Verification items for this drawing (mm, ordinates from the low corner). A direction names the side the tool comes from. Coordinates: 2 decimals unless noted, no trailing zeros. Order: outer loops, then holes, each group sorted by start corner. A loop starts at its lowest first (then second) coordinate and runs counter-clockwise, first axis right, second up. Notation, with made-up numbers: (-37.75, 13.5) -> (-13.75, 13.5) arc R19 ccw to (-13.75, 34.5) -> close; hole circle Ø9 at (-33, -40). An arc over 180 degrees is marked (long way). Write each question's results on one line, items separated by ' | '. Start each with the question number.
(1) Thickness scan on probe 1 along Y at (x, z) = (4.5, 7.7); probe 2 along X at (y, z) = (19, 7.7); probe 3 along Z at (x, y) = (2, 22.5). Record the ranges inside material, lowest first. Write a range as [from, to].
(2) Draft check along X on the marked faces 4, 5, 6 and 7. Enter one of: +X half, -X half, draft (parallel to the pull), parting line (faces both ways), or undercut.
(3) Cross-section at D-D on y = 19.75. Enter the section's corners in (x, z).
(4) Cross-section at C-C on z = 4.75. Enter the section's corners in (x, y), and give its area (3 significant figures).
(5) Cross-section at B-B on x = 30. Enter the section's corners in (y, z).
(6) Cross-section at A-A on z = 8. Enter the section's corners in (x, y), and give its area (3 significant figures).
(7) Go/stop test with flat-tipped pins: pin 1 (9 mm diameter, centred on x = 29.5, y = 18, fed in from -Z); pin 2 (10 mm diameter, centred on x = 11, y = 10.5, fed in from -Z); pin 3 (1.5 mm diameter, centred on y = 13.5, z = 5, fed in from +X). Record where each tip stops, or that it passes through.
(8) Set-up check for the marked faces 1, 2 and 3: record each of +Z, -Z, +X, -X, +Y, -Y from which the full face is reachable in a straight line by a thin tool's end or side.
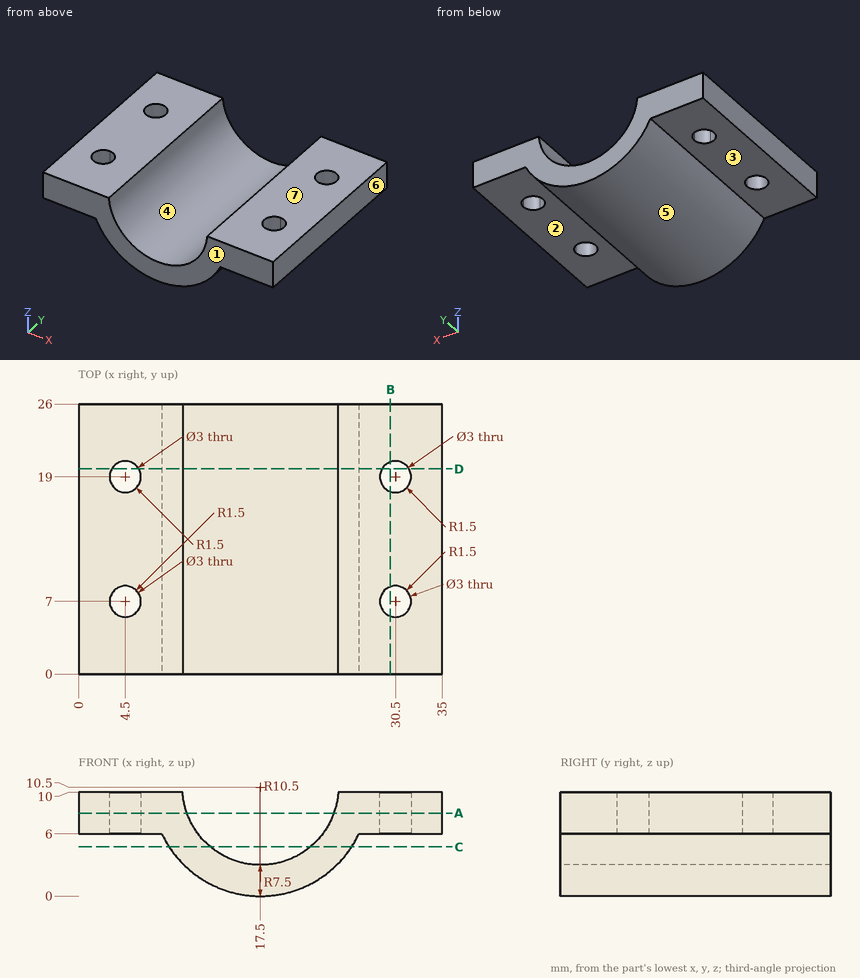
Results are:
1) probe 1: y = [0, 5.5], [8.5, 17.5], [20.5, 26] | probe 2: x = [0, 3], [6, 10.54], [24.46, 29], [32, 35] | probe 3: z = [6, 10]
2) face 4: undercut | face 5: parting line | face 6: +X half | face 7: draft
3) outline: (0, 6) -> (3.2, 6) -> (3.2, 10) -> (0, 10) -> close; (5.8, 6) -> (8.01, 6) arc R10.5 ccw to (26.99, 6) -> (29.2, 6) -> (29.2, 10) -> (24.98, 10) arc R7.5 cw to (10.02, 10) -> (5.8, 10) -> close; (31.8, 6) -> (35, 6) -> (35, 10) -> (31.8, 10) -> close
4) outline: (8.71, 0) -> (12.68, 0) -> (12.68, 26) -> (8.71, 26) -> close; (22.32, 0) -> (26.29, 0) -> (26.29, 26) -> (22.32, 26) -> close | area: 206 mm2
5) outline: (0, 6) -> (5.59, 6) -> (5.59, 10) -> (0, 10) -> close; (8.41, 6) -> (17.59, 6) -> (17.59, 10) -> (8.41, 10) -> close; (20.41, 6) -> (26, 6) -> (26, 10) -> (20.41, 10) -> close
6) outline: (0, 0) -> (10.43, 0) -> (10.43, 26) -> (0, 26) -> close; (24.57, 0) -> (35, 0) -> (35, 26) -> (24.57, 26) -> close; hole circle Ø3 at (4.5, 7); hole circle Ø3 at (4.5, 19); hole circle Ø3 at (30.5, 7); hole circle Ø3 at (30.5, 19) | area: 514 mm2
7) pin 1: stops at z = 3.15 | pin 2: stops at z = 0.11 | pin 3: stops at x = 26.86
8) face 1: +Z, -Z, +X, -X, -Y | face 2: -Z, +X, +Y, -Y | face 3: -Z, -X, +Y, -Y
